Source: CAD feature listing. Evaluate the final solid. Frame: model axes, mm. A direction names the side the tool comes from. Give positions to 0.01 mm unless a question says otherwise; leave off trailing zeros. Order: outer loops, then holes, each group sorted by start corner. A loop starts at its lowest first (then second) coordinate and runs counter-clockwise, first axis right, second up. Notation, with made-up numbers: M 6.5,56.25 L 10.5,56.25 A18 cw 10.5,64.25 Z; hole C 55,76.25 d10. An arc over 180 degrees is marked long. Answer in a Markdown table with one row per item. Add a question column.
(1) Set-up query: faces 4 (the face through (-40.41, 1.44, 84.62)), 5 (the face through (63.1, 1.4, 77.9)). Return all of +Z, -Z, +X, -X, +Y, -Y with unobstructed straight access to the full face (end or side cutting, diameter ignored); none if empty.
(2) Section query B-B, the plane z = 38.5. Return loops of the section in (x, y).
(3) Mould query, pull axis X, two halves, no side actions, for faces 1 (the face through (-63.1, 1.4, 77.9)), 2 (the face through (71.69, 1.44, 84.62)), 3 (the face through (-18, 0, -1)). Classes: pulls with the +X half, pulls with the -X half, needs draft (parallel to the pull), parting line crosses it, or undercut.
(4) Section query C-C, the plane x = 20.5. Return loops of the section in (y, z), plus the area to 3 significant figures.
(5) Material intervals for line 1 along X through (y, z) = (0.9, -63.9) (3 decimals); line 2 along X through (y, z) = (0.8, 0); line 3 along X through (y, z) = (1.1, 47.5), sorted ascending.
(6) Section query D-D, the plane y = 2.1. Count the separate pieces of the cut face and the enclosed holes in it, plus the area to 3 significant figures.
(7) Section query A-A, the plane x = 0. Return loops of the section in (y, z), plus the area to 3 significant figures.
(8) Pin query (flat end, axial travel): P1, Ø0.9, axis at x = -16, y = 2, coming from the +Z side; P2, Ø0.9, axis at y = 1, z = 61.5, coming from the +X side; P3, Ø1.4, axis at y = 1.5, z = -76.5, coming from the -X side. Return the tip coordinate at first contact, or that it passes through.
from build123d import *

# Parameters (mm, degrees)
SKETCH4_W               = 152.4
SKETCH4_H               = 177.8
BOSS_EXTRUDE2_DEPTH     = 2.85
SKETCH5_R               = 1.5
CUT_EXTRUDE1_DEPTH      = 118.122894858
SKETCH6_R               = 3
CUT_EXTRUDE2_DEPTH      = 118.122894858
SKETCH7_R               = 1.7
CUT_EXTRUDE3_DEPTH      = 118.122894858
SKETCH8_W               = 50
SKETCH8_H               = 50
CUT_EXTRUDE4_DEPTH      = 118.122894858
SKETCH9_R               = 1.7
SKETCH9_W               = 3
SKETCH9_H               = 10.5
CUT_EXTRUDE5_DEPTH      = 118.122894858
SKETCH10_W              = 71.8
SKETCH10_H              = 52.8
CUT_EXTRUDE6_DEPTH      = 118.122894858
SKETCH11_R              = 2.25
SKETCH11_W              = 42
SKETCH11_H              = 21
CUT_EXTRUDE7_DEPTH      = 118.122894858
SKETCH12_R              = 2
SKETCH12_R_2            = 0.8
CUT_EXTRUDE8_DEPTH      = 118.122894858
SKETCH13_R              = 1.85
CUT_EXTRUDE9_DEPTH      = 118.188619328
MIRROR3_COPY_1_SKETCH_R = 1.85
MIRROR3_COPY_1_DEPTH    = 118.188619328
FILLET1_R               = 15
FILLET2_R               = 15
SKETCH14_R              = 1.7
SKETCH14_W              = 2.85
SKETCH14_H              = 10
CUT_EXTRUDE10_DEPTH     = 118.122894858


with BuildPart() as part:
    # Sketch4 → Boss-Extrude2 (new body)
    with BuildSketch(Plane(origin=(0, 0, 0), x_dir=(1, 0, 0), z_dir=(0, 1, 0))):
        Rectangle(SKETCH4_W, SKETCH4_H)
    extrude(amount=BOSS_EXTRUDE2_DEPTH)

    # Sketch5 → Cut-Extrude1 (cut, through all)
    with BuildSketch(Plane.XZ):
        with Locations(Location((0, -63.9, 0), (0, 0, 270))):
            Circle(SKETCH5_R)
    extrude(amount=-CUT_EXTRUDE1_DEPTH, mode=Mode.SUBTRACT)

    # Sketch6 → Cut-Extrude2 (cut, through all)
    with BuildSketch(Plane(origin=(0, 2.85, 0), x_dir=(1, 0, 0), z_dir=(0, 1, 0))):
        with Locations(Location((0, 0, 0), (0, 0, 270))):
            Circle(SKETCH6_R)
    extrude(amount=-CUT_EXTRUDE2_DEPTH, mode=Mode.SUBTRACT)

    # Sketch7 → Cut-Extrude3 (cut, through all)
    with BuildSketch(Plane.XZ):
        with Locations(Location((37.5, 0, 0), (0, 0, 270))):
            Circle(SKETCH7_R)
        with Locations(Location((-37.5, 0, 0), (0, 0, 270))):
            Circle(SKETCH7_R)
    extrude(amount=-CUT_EXTRUDE3_DEPTH, mode=Mode.SUBTRACT)

    # Sketch8 → Cut-Extrude4 (cut, through all)
    with BuildSketch(Plane.XZ):
        with Locations((0, -63.9)):
            Rectangle(SKETCH8_W, SKETCH8_H)
    extrude(amount=-CUT_EXTRUDE4_DEPTH, mode=Mode.SUBTRACT)

    # Sketch9 → Cut-Extrude5 (cut, through all)
    with BuildSketch(Plane(origin=(0, 2.85, 0), x_dir=(1, 0, 0), z_dir=(0, 1, 0))):
        with Locations(Location((-64.2, -63.9, 0), (0, 0, 270))):
            Circle(SKETCH9_R)
        with Locations((-74.7, -63.9)):
            Rectangle(SKETCH9_W, SKETCH9_H)
    cut_extrude5 = extrude(amount=-CUT_EXTRUDE5_DEPTH, mode=Mode.SUBTRACT)

    # Sketch10 → Cut-Extrude6 (cut, through all)
    with BuildSketch(Plane.XZ):
        with Locations((0, 62.5)):
            Rectangle(SKETCH10_W, SKETCH10_H)
    extrude(amount=-CUT_EXTRUDE6_DEPTH, mode=Mode.SUBTRACT)

    # Sketch11 → Cut-Extrude7 (cut, through all)
    with BuildSketch(Plane.XZ):
        with Locations(Location((-14.85, -23.85, 0), (0, 0, 270))):
            Circle(SKETCH11_R)
        with Locations(Location((-14.85, -33.95, 0), (0, 0, 270))):
            Circle(SKETCH11_R)
        with Locations(Location((33.25, -33.95, 0), (0, 0, 270))):
            Circle(SKETCH11_R)
        with Locations(Location((33.25, -23.85, 0), (0, 0, 270))):
            Circle(SKETCH11_R)
        with Locations((9.2, -28.9)):
            Rectangle(SKETCH11_W, SKETCH11_H)
    extrude(amount=-CUT_EXTRUDE7_DEPTH, mode=Mode.SUBTRACT)

    # Sketch12 → Cut-Extrude8 (cut, through all)
    with BuildSketch(Plane.XZ):
        with Locations(Location((0, 22.5, 0), (0, 0, 270))):
            Circle(SKETCH12_R)
        with Locations(Location((-4.5, 22.5, 0), (0, 0, 270))):
            Circle(SKETCH12_R_2)
        with Locations(Location((4.5, 22.5, 0), (0, 0, 270))):
            Circle(SKETCH12_R_2)
    extrude(amount=-CUT_EXTRUDE8_DEPTH, mode=Mode.SUBTRACT)

    # Sketch13 → Cut-Extrude9 (cut, through all)
    with BuildSketch(Plane(origin=(0, 4.85, 0), x_dir=(1, 0, 0), z_dir=(0, 1, 0))):
        with Locations(Location((-63.7, -76.15, 0), (0, 0, 270))):
            Circle(SKETCH13_R)
        with Locations(Location((-47.7, -76.15, 0), (0, 0, 270))):
            Circle(SKETCH13_R)
    cut_extrude9 = extrude(amount=-CUT_EXTRUDE9_DEPTH, mode=Mode.SUBTRACT)

    # Mirror1: Cut-Extrude5 across plane
    add(cut_extrude5.mirror(Plane(origin=(0, 0, 0), x_dir=(0, 0, 1), z_dir=(1, 0, 0))), mode=Mode.SUBTRACT)

    # Mirror2: Cut-Extrude9 across plane
    add(cut_extrude9.mirror(Plane.XY), mode=Mode.SUBTRACT)

    # Mirror3: Cut-Extrude9 across plane
    add(cut_extrude9.mirror(Plane(origin=(0, 0, 0), x_dir=(0, 0, 1), z_dir=(1, 0, 0))), mode=Mode.SUBTRACT)

    # Mirror3 copy 1 sketch → Mirror3 copy 1 (cut, through all)
    with BuildSketch(Plane(origin=(0, 4.85, 0), x_dir=(-1, 0, 0), z_dir=(0, 1, 0))):
        with Locations(Location((-63.7, -76.15, 0), (0, 0, 270))):
            Circle(MIRROR3_COPY_1_SKETCH_R)
        with Locations(Location((-47.7, -76.15, 0), (0, 0, 270))):
            Circle(MIRROR3_COPY_1_SKETCH_R)
    extrude(amount=-MIRROR3_COPY_1_DEPTH, mode=Mode.SUBTRACT)

    # Fillet1
    fillet1_edges = [part.edges().sort_by_distance(p)[0] for p in [
        (76.2, 1.425, 88.9),
        (-76.2, 1.425, 88.9),
        (-76.2, 1.425, -88.9),
        (76.2, 1.425, -88.9),
    ]]
    fillet(fillet1_edges, radius=FILLET1_R)

    # Fillet2
    fillet2_edges = [part.edges().sort_by_distance(p)[0] for p in [
        (25, 1.425, -88.9),
        (-25, 1.425, -88.9),
        (-35.9, 1.425, 88.9),
        (35.9, 1.425, 88.9),
    ]]
    fillet(fillet2_edges, radius=FILLET2_R)

    # Sketch14 → Cut-Extrude10 (cut, through all)
    with BuildSketch(Plane.XZ):
        with Locations(Location((40.575, -63.9, 0), (0, 0, 270))):
            Circle(SKETCH14_R)
        with Locations((40.575, -78.9)):
            Rectangle(SKETCH14_W, SKETCH14_H)
        with Locations((40.575, -48.9)):
            Rectangle(SKETCH14_W, SKETCH14_H)
    cut_extrude10 = extrude(amount=-CUT_EXTRUDE10_DEPTH, mode=Mode.SUBTRACT)

    # Mirror4: Cut-Extrude10 across plane
    add(cut_extrude10.mirror(Plane(origin=(0, 0, 0), x_dir=(0, 0, 1), z_dir=(1, 0, 0))), mode=Mode.SUBTRACT)


solid = part.part
Values follow:
| question | item | result |
|---|---|---|
| 1 | face 4 | +Z, +Y, -Y |
| 1 | face 5 | +Y, -Y |
| 2 | outline | M -76.2,0 L -35.9,0 L -35.9,2.85 L -76.2,2.85 Z; M 35.9,0 L 76.2,0 L 76.2,2.85 L 35.9,2.85 Z |
| 3 | face 1 | undercut |
| 3 | face 2 | pulls with the +X half |
| 3 | face 3 | needs draft |
| 4 | outline | M 0,-18.4 L 2.85,-18.4 L 2.85,36.1 L 0,36.1 Z |
| 4 | area | 155 mm² |
| 5 | line 1 | x = -76.2 to -42.275, -38.875 to -25, 25 to 38.875, 42.275 to 76.2 |
| 5 | line 2 | x = -76.2 to -39.2, -35.8 to -3, 3 to 35.8, 39.2 to 76.2 |
| 5 | line 3 | x = -76.2 to -35.9, 35.9 to 76.2 |
| 6 | separate pieces | 1 |
| 6 | enclosed holes | 26 |
| 6 | area | 19,100 mm² |
| 7 | outline | M 0,-18.4 L 2.85,-18.4 L 2.85,-3 L 0,-3 Z; M 0,3 L 2.85,3 L 2.85,20.5 L 0,20.5 Z; M 0,24.5 L 2.85,24.5 L 2.85,36.1 L 0,36.1 Z |
| 7 | area | 127 mm² |
| 8 | P1 | stops at z = 36.1 |
| 8 | P2 | stops at x = 73.2 |
| 8 | P3 | stops at x = -76.08 |
